from build123d import *

# Parameters (mm, degrees)
SKETCH1_R                = 2.75
BOSS_EXTRUDE1_DEPTH      = 2
SKETCH2_W                = 3
SKETCH2_H                = 100
BOSS_EXTRUDE2_DEPTH      = 2
SKETCH3_W                = 60
SKETCH3_H                = 3
BOSS_EXTRUDE3_DEPTH      = 2
CHAMFER1_SIZE            = 2
CHAMFER1_OF_MIRROR1_SIZE = 2
CUT_EXTRUDE2_DEPTH       = 122.80201158
CUT_EXTRUDE2_DEPTH_BACK  = 122.80201158
CUT_EXTRUDE3_DEPTH       = 116.034690529
CUT_EXTRUDE3_DEPTH_BACK  = 116.034690529
SKETCH5_R                = 2.6


with BuildPart() as part:
    # Sketch1 → Boss-Extrude1 (new body)
    with BuildSketch(Plane(origin=(0, 0, 0), x_dir=(1, 0, 0), z_dir=(0, 1, 0))):
        Polygon((-17.5, 42.995), (-17.5, -42.995), (-36.7, -42.995), (-36.7, -109.005), (36.7, -109.005), (36.7, -42.995), (17.5, -42.995), (17.5, 42.995), (36.7, 42.995), (36.7, 109.005), (-36.7, 109.005), (-36.7, 42.995), align=None)
        with Locations(Location((-31.7, 102.855, 0), (0, 0, 270))):
            Circle(SKETCH1_R, mode=Mode.SUBTRACT)
        with Locations(Location((-31.7, 49.145, 0), (0, 0, 270))):
            Circle(SKETCH1_R, mode=Mode.SUBTRACT)
        with Locations(Location((31.7, 49.145, 0), (0, 0, 270))):
            Circle(SKETCH1_R, mode=Mode.SUBTRACT)
        with Locations(Location((31.7, 102.855, 0), (0, 0, 270))):
            Circle(SKETCH1_R, mode=Mode.SUBTRACT)
        with Locations(Location((31.7, -102.855, 0), (0, 0, 270))):
            Circle(SKETCH1_R, mode=Mode.SUBTRACT)
        with Locations(Location((31.7, -49.145, 0), (0, 0, 270))):
            Circle(SKETCH1_R, mode=Mode.SUBTRACT)
        with Locations(Location((-31.7, -49.145, 0), (0, 0, 270))):
            Circle(SKETCH1_R, mode=Mode.SUBTRACT)
        with Locations(Location((-31.7, -102.855, 0), (0, 0, 270))):
            Circle(SKETCH1_R, mode=Mode.SUBTRACT)
    extrude(amount=BOSS_EXTRUDE1_DEPTH)

    # Sketch2 → Boss-Extrude2 (add)
    with BuildSketch(Plane(origin=(0, 2, 0), x_dir=(1, 0, 0), z_dir=(0, 1, 0))):
        with Locations((12, -50)):
            Rectangle(SKETCH2_W, SKETCH2_H)
        with Locations((0, -50)):
            Rectangle(SKETCH2_W, SKETCH2_H)
        with Locations((-12, -50)):
            Rectangle(SKETCH2_W, SKETCH2_H)
    boss_extrude2 = extrude(amount=BOSS_EXTRUDE2_DEPTH)

    # Sketch3 → Boss-Extrude3 (add)
    with BuildSketch(Plane(origin=(0, 2, 0), x_dir=(1, 0, 0), z_dir=(0, 1, 0))):
        with Locations((0, -91)):
            Rectangle(SKETCH3_W, SKETCH3_H)
        with Locations((0, -61)):
            Rectangle(SKETCH3_W, SKETCH3_H)
        with Locations((0, -76)):
            Rectangle(SKETCH3_W, SKETCH3_H)
    boss_extrude3 = extrude(amount=BOSS_EXTRUDE3_DEPTH)

    # Chamfer1
    chamfer1_edges = [part.edges().sort_by_distance(p)[0] for p in [
        (30, 4, 61),
        (30, 4, 76),
        (30, 4, 91),
        (12, 4, 100),
        (0, 4, 100),
        (-12, 4, 100),
        (-30, 4, 91),
        (-30, 4, 76),
        (-30, 4, 61),
    ]]
    chamfer(chamfer1_edges, length=CHAMFER1_SIZE - 0.0001)  # a hair under: the kernel refuses the full size

    # Mirror1: Boss-Extrude2, Boss-Extrude3 across plane
    add(boss_extrude2.mirror(Plane.XY))
    add(boss_extrude3.mirror(Plane.XY))

    # Chamfer1 of Mirror1
    chamfer1_of_mirror1_edges = [part.edges().sort_by_distance(p)[0] for p in [
        (30, 4, -61),
        (30, 4, -76),
        (30, 4, -91),
        (12, 4, -100),
        (0, 4, -100),
        (-12, 4, -100),
        (-30, 4, -91),
        (-30, 4, -76),
        (-30, 4, -61),
    ]]
    chamfer(chamfer1_of_mirror1_edges, length=CHAMFER1_OF_MIRROR1_SIZE - 0.0001)  # a hair under: the kernel refuses the full size

    # Sketch4 → Cut-Extrude2 (cut, two sides: drawn at the far end of the back side and taken through both)
    with BuildSketch(Plane(origin=(17.5, 0, 0), x_dir=(0, 0, -1), z_dir=(1, 0, 0)).offset(-CUT_EXTRUDE2_DEPTH_BACK)):
        Polygon((13, 0), (13, 2), (-15, 2), (-15, 4), (109.005, 4), (109.005, 0), align=None)
    extrude(amount=CUT_EXTRUDE2_DEPTH + CUT_EXTRUDE2_DEPTH_BACK, mode=Mode.SUBTRACT)

    # Sketch5 → Cut-Extrude3 (cut, two sides: drawn at the far end of the back side and taken through both)
    with BuildSketch(Plane(origin=(0, 2, 0), x_dir=(1, 0, 0), z_dir=(0, 1, 0)).offset(-CUT_EXTRUDE3_DEPTH_BACK)):
        with Locations(Location((10, -8, 0), (0, 0, 270))):
            Circle(SKETCH5_R)
        with Locations(Location((10, 8, 0), (0, 0, 270))):
            Circle(SKETCH5_R)
        with Locations(Location((-10, 8, 0), (0, 0, 270))):
            Circle(SKETCH5_R)
        with Locations(Location((-10, -8, 0), (0, 0, 270))):
            Circle(SKETCH5_R)
    extrude(amount=CUT_EXTRUDE3_DEPTH + CUT_EXTRUDE3_DEPTH_BACK, mode=Mode.SUBTRACT)


solid = part.part
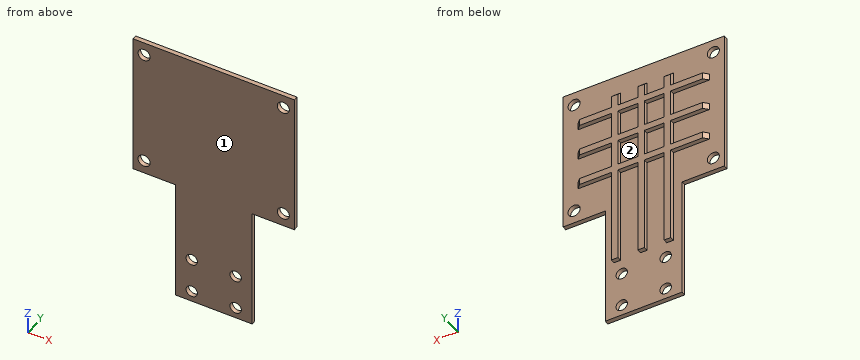
Check sheet for the modelled part. Datum: model origin and axes. Units: mm. Face numbers are marked on the shaded views. Round coordinates to 2 decimals unless told otherwise and drop trailing zeros. Loops run counter-clockwise (first coordinate to the right, second up) from the corner with the lowest first, then second, coordinate; pieces in that order, holes last. Notation, with made-up numbers: M 55.5,0.25 L 66.5,0.25 A29 ccw 66.5,27.25 Z; hole C 53,31.25 d10. An arc over 180 degrees is marked long. One line per question, with ' | ' between items. Start each with the question number.
Item 1: Gauge pin test, flat ends, axial feed: pin 1 Ø2 at (y, z) = (0.5, 24) entering from -X; pin 2 Ø2 at (y, z) = (3.5, 69.5) entering from +X; pin 3 Ø1.6 at (x, y) = (-25.5, 3) entering from +Z. Record the tip position at first contact, or that the pin passes through.
Item 2: Section check A-A (z = -8). Record the boundary of the cut face in (x, y).
Item 3: Section check C-C (x = -31.7). Record the boundary of the cut face in (y, z) (3 decimals).
Item 4: Release check for a two-part mould opening along Z. For the marked faces 1 and 2 record: released by +Z, released by -Z, zero draft, split by the parting line, or undercut.
Item 5: Section check B-B (y = 1.25). State how many separate pieces and enclosed holes the cut face has, and give its area (3 significant figures).
Item 6: Section check D-D (x = -20). Record the boundary of the cut face in (y, z) (3 decimals).
Item 7: Scan lines: probe 1 along Z at (x, y) = (10, 0.55) (3 decimals); probe 2 along X at (y, z) = (2.3, 15.5); probe 3 along Z at (x, y) = (18, 2.5). Record each from-to range of solid material in increasing order.
Worked out:
1) pin 1: x = -17.5 | pin 2: x = 13.5 | pin 3: z = 92.5
2) outline: M -17.5,0 L -12.6,0 L -12.6,2 L -17.5,2 Z; M -7.4,0 L 7.4,0 L 7.4,2 L -7.4,2 Z; M 12.6,0 L 17.5,0 L 17.5,2 L 12.6,2 Z
3) outline: M 0,42.995 L 2,42.995 L 2,46.395 L 0,46.395 Z; M 0,51.895 L 2,51.895 L 2,100.105 L 0,100.105 Z; M 0,105.605 L 2,105.605 L 2,109.005 L 0,109.005 Z
4) face 1: zero draft | face 2: undercut
5) separate pieces: 1 | enclosed holes: 8 | area: 6,620 mm^2
6) outline: M 0,42.995 L 2,42.995 L 2,59.5 L 4,59.5 L 4,62.5 L 2,62.5 L 2,74.5 L 4,74.5 L 4,77.5 L 2,77.5 L 2,89.5 L 4,89.5 L 4,92.5 L 2,92.5 L 2,109.005 L 0,109.005 Z
7) probe 1: -13 to -10.6, -5.4 to 5.4, 10.6 to 109.005 | probe 2: -13.5 to -10.5, -1.5 to 1.5, 10.5 to 13.5 | probe 3: 59.5 to 62.5, 74.5 to 77.5, 89.5 to 92.5
